Source: CAD feature listing. Evaluate the final solid. Frame: model axes, mm. A direction names the side the tool comes from. Round coordinates to 2 decimals unless told otherwise and drop trailing zeros. Loops run counter-clockwise (first coordinate to the right, second up) from the corner with the lowest first, then second, coordinate; pieces in that order, holes last. Notation, with made-up numbers: (-38, -24.75) - (-3, -24.75) arc R20 ccw to (-3, -13.75) - close; hole circle Ø2 at (56.25, -6.5). An arc over 180 degrees is marked (long way). One line per question, with ' | ' between items. Start each with the question number.
1. Cut plane B-B (z = -247). Return loops of the section in (x, y).
2. Ray query, line 1 (X direction, y = 0, z = -156); line 2 (Z direction, x = 0, y = 0); line 3 (Z direction, x = 6, y = -6). Return the intervals inside material, ascending.
3. Access query for faces 1 (the flat face through (0, 7, -120)), 2 (the flat face through (0, 0, 0)), 3 (the flat face through (0, 7, -123)). Directions: +Z, -Z, +X, -X, +Y, -Y. A direction counts if a zero-diameter tool reaches every point of the face in a straight line with its end or side. Return the directions, or none.
4. Cut plane A-A (y = 0). Return loops of the section in (x, z).
5. Pin query (flat end, axial travel): pin 1 (12 mm diameter, centred on x = 5, z = -236.5, fed in from -Y); pin 2 (5 mm diameter, centred on x = -8.5, y = -4.5, fed in from +Z); pin 3 (1 mm diameter, centred on x = 2.5, z = -168.5, fed in from -Y); pin 4 (3 mm diameter, centred on x = 12.5, y = -13, fed in from +Z). Return the tip coordinate at first contact, or that it passes through.
Autodesk Inventor part; units mm, degrees
ref_plane "YZ Plane" through (0, 0, 0) normal (1, 0, 0) x (0, 1, 0)
ref_plane "XZ Plane" through (0, 0, 0) normal (0, 1, 0) x (-1, 0, 0)
ref_plane "XY Plane" through (0, 0, 0) normal (0, 0, 1) x (1, 0, 0)
sketch "Sketch1" plane through (0, 0, 0) normal (0, 1, 0) x (-1, 0, 0)
  line L0 (0, 0) -> (6, 0)
  line L1 (6, 0) -> (6, -120)
  line L2 (6, -120) -> (16, -120)
  line L3 (16, -120) -> (16, -123)
  line L4 (16, -123) -> (6, -123)
  line L5 (6, -123) -> (6, -273)
  line L6 (6, -273) -> (0, -273)
  line L7 (0, -273) -> (0, 0)
  dimension "d0" = 120
  dimension "d1" = 3
  dimension "d2" = 10
  dimension "d3" = 150
  dimension "d4" = 6
revolve "Revolution1" add sketch "Sketch1" angle 360 about axis through (0, 0, -273) along (0, 0, 1)
sketch "Sketch3" plane through (0, 0, 0) normal (0, 1, 0) x (-1, 0, 0)
  circle A0 centre (0, -156) radius 1.5
  line L0 (-16, -123) -> (16, -123)
  point P0 (0, 0)
  dimension "d6" = 3
  dimension "d7" = 33
extrude "Extrusion1" cut sketch "Sketch3" along normal through all both and the other way through all
chamfer "Chamfer1" distance 2 angle 45 2 edges at (6, 0, -273) (6, 0, 0)
chamfer "Chamfer2" distance 0.5 angle 45 2 edges at (16, 0, -123) (16, 0, -120)
properties part number "Handle"
Answers follow:
1) outline: circle Ø12 at (0, 0)
2) line 1: x = -6 to -1.5, 1.5 to 6 | line 2: z = -273 to -157.5, -154.5 to 0 | line 3: z = -123 to -120
3) face 1: +Z | face 2: +Z, +X, -X, +Y, -Y | face 3: -Z
4) outline: (-16, -122.5) - (-15.5, -123) - (-6, -123) - (-6, -271) - (-4, -273) - (4, -273) - (6, -271) - (6, -123) - (15.5, -123) - (16, -122.5) - (16, -120.5) - (15.5, -120) - (6, -120) - (6, -2) - (4, 0) - (-4, 0) - (-6, -2) - (-6, -120) - (-15.5, -120) - (-16, -120.5) - close; hole circle Ø3 at (0, -156)
5) pin 1: stops at y = -6 | pin 2: stops at z = -120 | pin 3: stops at y = -5.66 | pin 4: passes through
